Work out the finished part from the listing and answer in its coordinate system (mm). A direction names the side the tool comes from. Round coordinates to 2 decimals unless told otherwise and drop trailing zeros. Order: outer loops, then holes, each group sorted by start corner. A loop starts at its lowest first (then second) coordinate and runs counter-clockwise, first axis right, second up. Notation, with made-up numbers: (-28, 14.25) -> (-4, 14.25) arc R34 cw to (-4, 49.25) -> close; hole circle Ø5 at (-4, 87). An arc over 180 degrees is marked (long way). Use one line per item in the form item = value.
```python
from build123d import *

# Parameters (mm, degrees)
CUT_EXTRUDE1_DEPTH = 2.5


with BuildPart() as part:
    # Sketch1 → Revolve1 (revolve)
    with BuildSketch(Plane(origin=(0, 0, 0), x_dir=(0, 0, -1), z_dir=(1, 0, 0)), mode=Mode.PRIVATE) as revolve1_sk:
        Polygon((-23, 7.5), (-23, 14), (-9, 14), (-9, 45), (9, 45), (9, 14), (12, 14), (12, 7.5), align=None)
    revolve(revolve1_sk.sketch.rotate(Axis((0, 0, 42.784), (0, 0, -1)), 90), axis=Axis((0, 0, 42.784), (0, 0, -1)))

    # Sketch2 → Cut-Extrude1 (cut, symmetric)
    with BuildSketch(Plane(origin=(0, 0, 0), x_dir=(0, 0, -1), z_dir=(1, 0, 0))):
        Polygon((-23, 9.65), (-23, 5), (12, 5), (12, 10), align=None)
    extrude(amount=CUT_EXTRUDE1_DEPTH, both=True, mode=Mode.SUBTRACT)


solid = part.part
```
Item 1: The part is cut by section A-A, the plane y = 0. Give the vertices of the cut face in (x, z).
Findings:
outline = (-45, -9) -> (-14, -9) -> (-14, -12) -> (-7.5, -12) -> (-7.5, 23) -> (-14, 23) -> (-14, 9) -> (-45, 9) -> close; (7.5, -12) -> (14, -12) -> (14, -9) -> (45, -9) -> (45, 9) -> (14, 9) -> (14, 23) -> (7.5, 23) -> close
Item 2: The part is cut by section B-B, the plane x = 0. Give the vertices of the cut face in (y, z).
Findings:
outline = (-45, -9) -> (-14, -9) -> (-14, -12) -> (-7.5, -12) -> (-7.5, 23) -> (-14, 23) -> (-14, 9) -> (-45, 9) -> close; (9.65, 23) -> (10, -12) -> (14, -12) -> (14, -9) -> (45, -9) -> (45, 9) -> (14, 9) -> (14, 23) -> close
Item 3: Determine the mould class of faces 4 (the cylindrical face through (0.294, -7.494, 5.745)), 5 (the cylindrical face through (20.765, 39.923, -0.126)), 6 (the flat face through (9, -11, -9)) for opening direction Y: released by +Y, released by -Y, zero draft, split by the parting line, or undercut.
Findings:
face_4 = undercut
face_5 = split by the parting line
face_6 = zero draft
Item 4: Flat-ended cylindrical pins translate along their axes: P1, Ø4, axis at x = -1, z = 8.5, coming from the +Y side; P2, Ø10, axis at x = -3.5, y = 30.5, coming from the +Z side; P3, Ø5, axis at y = 10.5, z = 1, coming from the -X side; P4, Ø1, axis at x = -36, y = -30.5, coming from the -Z side. Find the tip coordinate at first contact, or state that the pin passes through.
Findings:
P1 = 45
P2 = 9
P3 = -44.28
P4 = through
Item 5: Consider line 1 along Z through (x, y) = (29, 8); line 2 along Y through (x, z) = (0, 10); line 3 along Y through (x, z) = (-30, -1). Determine where each line is inside the solid, lowest interval first.
Findings:
line_1 = -9 to 9
line_2 = -14 to -7.5, 9.78 to 14
line_3 = -33.54 to 33.54
Item 6: For faces 1 (the flat face through (-9, -11, 9)), 2 (the cylindrical face through (6.5, 12.4, -10.5)), 3 (the flat face through (-6, 6, 23)), determine the directions among +Z, -Z, +X, -X, +Y, -Y from which every point of the face is accessible in a straight line to the end or side of a thin tool.
Findings:
face_1 = +Z
face_2 = -Z
face_3 = +Z, +X, -X, +Y, -Y
Item 7: The part is cut by section C-C, the plane z = -1. Give the vertices of the cut face in (x, y).
Findings:
outline = circle Ø90 at (0, 0); hole (-2.5, 7.07) arc R7.5 ccw (long way) to (2.5, 7.07) -> (2.5, 9.89) -> (-2.5, 9.89) -> close
Item 8: The part is cut by section D-D, the plane z = 11. Give the vertices of the cut face in (x, y), and give its area (3 significant figures).
Findings:
outline = circle Ø28 at (0, 0); hole (-2.5, 7.07) arc R7.5 ccw (long way) to (2.5, 7.07) -> (2.5, 9.77) -> (-2.5, 9.77) -> close
area = 427 mm^2
